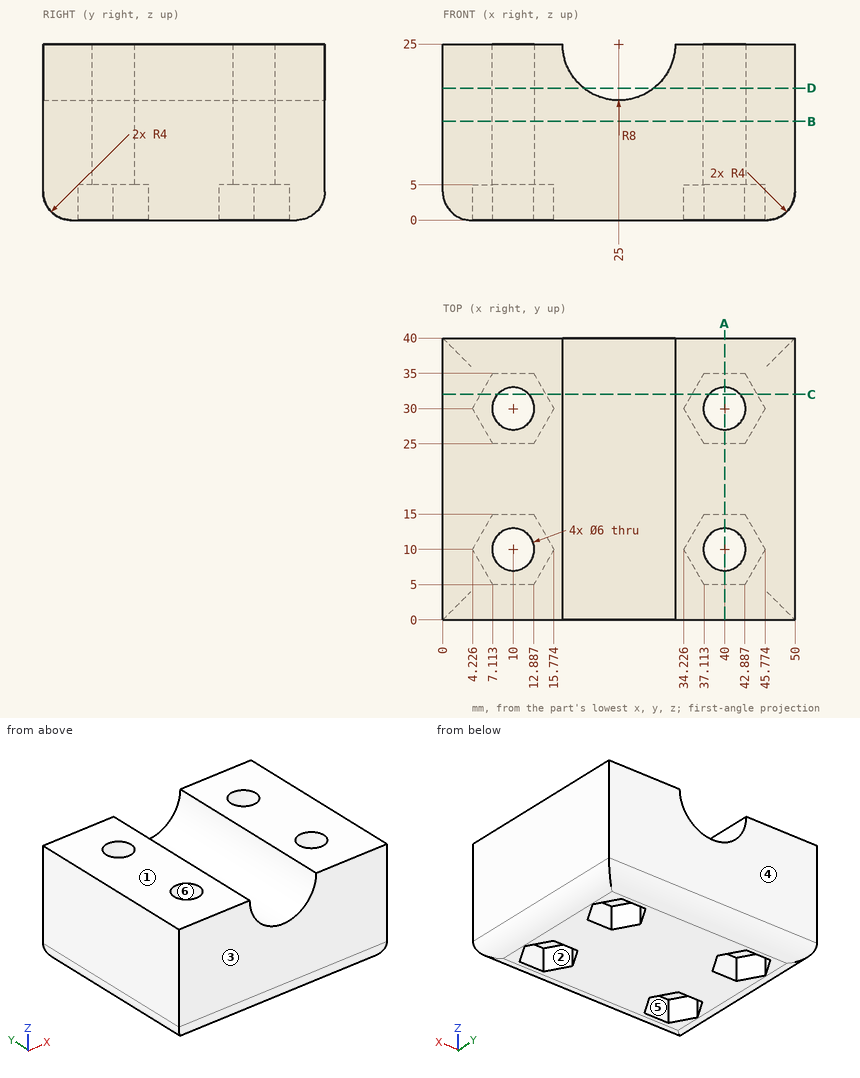
Here's the drawing with two shaded views (mm, measured from the low corner). I have some questions. A direction names the side the tool comes from. Give positions to 0.01 mm unless a question says otherwise; leave off trailing zeros. Order: outer loops, then holes, each group sorted by start corner. A loop starts at its lowest first (then second) coordinate and runs counter-clockwise, first axis right, second up. Notation, with made-up numbers: (84, 89.25) -> (122, 89.25) arc R18 ccw to (122, 121.25) -> close; hole circle Ø5 at (1, 79.25). An arc over 180 degrees is marked (long way). Use a Markdown table: item, result. Add a question column.
Item 1: Imagine slicing it at C-C on y = 32. Please give me the cut outline in (x, z).
Item 2: Imagine slicing it at B-B on z = 14. Please give me the cut outline in (x, y), plus the area to 3 significant figures.
Item 3: For the marked faces 5 and 6, which set-ups out of +Z, -Z, +X, -X, +Y, -Y let a thin tool reach every point of the face, with its end or its side?
Item 4: Imagine slicing it at A-A on x = 40. Please give me the cut outline in (y, z), plus the area to 3 significant figures.
Item 5: If we mould it in two halves opening along Y, with no side actions, what happens to the marked faces 1, 2, 3 and 4? For each: pulls with the +Y half, pulls with the -Y half, needs draft (parallel to the pull), parting line crosses it, or undercut.
Item 6: I need wall thicknesses on line 1 (Y direction, x = 10, z = 14); line 2 (X direction, y = 12, z = 4.25); line 3 (Z direction, x = 25, y = 16.5). Which ranges of each line are inside material? Lowest first, please.
Item 7: Imagine slicing it at D-D on z = 18.75. Please give me the cut outline in (x, y).
Item 8: Will these pins go through, and if not, where does the flat tip stop? pin 1 (8 mm diameter, centred on x = 26, y = 16.5, fed in from +Z) (1 decimal); pin 2 (10 mm diameter, centred on x = 24, y = 21, fed in from +Z); pin 3 (1.5 mm diameter, centred on x = 41.5, z = 2.5, fed in from -Y).
Data:
| question | item | result |
|---|---|---|
| 1 | outline | (0, 4) arc R4 ccw to (4, 0) -> (5.38, 0) -> (5.38, 5) -> (7.76, 5) -> (7.76, 25) -> (0, 25) -> close; (12.24, 5) -> (14.62, 5) -> (14.62, 0) -> (35.38, 0) -> (35.38, 5) -> (37.76, 5) -> (37.76, 25) -> (33, 25) arc R8 cw to (17, 25) -> (12.24, 25) -> close; (42.24, 5) -> (44.62, 5) -> (44.62, 0) -> (46, 0) arc R4 ccw to (50, 4) -> (50, 25) -> (42.24, 25) -> close |
| 2 | outline | (0, 0) -> (50, 0) -> (50, 40) -> (0, 40) -> close; hole circle Ø6 at (10, 10); hole circle Ø6 at (10, 30); hole circle Ø6 at (40, 10); hole circle Ø6 at (40, 30) |
| 2 | area | 1,890 mm² |
| 3 | face 5 | -Z |
| 3 | face 6 | +Z, -Z |
| 4 | outline | (0, 4) arc R4 ccw to (4, 0) -> (5, 0) -> (5, 5) -> (7, 5) -> (7, 25) -> (0, 25) -> close; (13, 5) -> (15, 5) -> (15, 0) -> (25, 0) -> (25, 5) -> (27, 5) -> (27, 25) -> (13, 25) -> close; (33, 5) -> (35, 5) -> (35, 0) -> (36, 0) arc R4 ccw to (40, 4) -> (40, 25) -> (33, 25) -> close |
| 4 | area | 653 mm² |
| 5 | face 1 | needs draft |
| 5 | face 2 | undercut |
| 5 | face 3 | pulls with the -Y half |
| 5 | face 4 | pulls with the +Y half |
| 6 | line 1 | y = 0 to 7, 13 to 27, 33 to 40 |
| 6 | line 2 | x = 0 to 5.38, 14.62 to 35.38, 44.62 to 50 |
| 6 | line 3 | z = 0 to 17 |
| 7 | outline | (0, 0) -> (20.01, 0) -> (20.01, 40) -> (0, 40) -> close; (29.99, 0) -> (50, 0) -> (50, 40) -> (29.99, 40) -> close; hole circle Ø6 at (10, 10); hole circle Ø6 at (10, 30); hole circle Ø6 at (40, 10); hole circle Ø6 at (40, 30) |
| 8 | pin 1 | stops at z = 18.8 |
| 8 | pin 2 | stops at z = 19.71 |
| 8 | pin 3 | stops at y = 0.07 |
